The model under review builds one solid part; all positions refer to its coordinate system, in mm. A direction names the side the tool comes from. Coordinates: 2 decimals unless noted, no trailing zeros. Order: outer loops, then holes, each group sorted by start corner. A loop starts at its lowest first (then second) coordinate and runs counter-clockwise, first axis right, second up.
```python
from build123d import *

# Parameters (mm, degrees)
EXTRUDE_1_DEPTH     = 500
CUT_EXTRUDE_1_DEPTH = 165
SKETCH_4_R          = 20
SKETCH_4_R_2        = 9.341042427
SKETCH_4_R_3        = 10
EXTRUDE_2_DEPTH     = 30
SKETCH_5_R          = 8.254931616
SKETCH_5_R_2        = 9.226679221
EXTRUDE_3_DEPTH     = 30


with BuildPart() as part:
    # Эскиз2 → Бобышка-Вытянуть1 (new body)
    with BuildSketch(Plane.XY):
        with BuildLine():
            Line((-164, 0), (164, 0))
            Line((164, 0), (164, 281.346442364))
            ThreePointArc((164, 281.346442364), (158.142135624, 295.488577987), (144, 301.346442364))
            Line((144, 301.346442364), (128.648418925, 301.346442364))
            Line((128.648418925, 301.346442364), (102.483646542, 329.199264578))
            Line((102.483646542, 329.199264578), (-102.483646542, 329.199264578))
            Line((-102.483646542, 329.199264578), (-128.648418925, 301.346442364))
            Line((-128.648418925, 301.346442364), (-144, 301.346442364))
            ThreePointArc((-144, 301.346442364), (-158.142135624, 295.488577987), (-164, 281.346442364))
            Line((-164, 281.346442364), (-164, 0))
        make_face()
    extrude(amount=EXTRUDE_1_DEPTH)

    # Эскиз3 → Вырез-Вытянуть1 (cut, symmetric)
    with BuildSketch(Plane(origin=(0, 0, 0), x_dir=(0, 0, -1), z_dir=(1, 0, 0))):
        Polygon((-463.138471818, 344.733431976), (-500, 301.346442364), (-514.613262102, 301.346442364), (-514.613262102, 363.370856045), (0, 363.370856045), (0, 301.346442364), (-40.69019293, 344.733431976), (-73.527559146, 339.458620278), (-40.69019293, 301.346442364), (-469.350946507, 301.346442364), (-431.238768593, 339.458620278), align=None)
    extrude(amount=CUT_EXTRUDE_1_DEPTH, both=True, mode=Mode.SUBTRACT)

    # Эскиз4 → Бобышка-Вытянуть2 (add)
    with BuildSketch(Plane.XY.offset(500)):
        with Locations((-110, 47.069313646)):
            Circle(SKETCH_4_R)
        with Locations((-60, 47.069313646)):
            Circle(SKETCH_4_R_2)
        with Locations((110.509329497, 47.069313646)):
            Circle(SKETCH_4_R)
        with Locations((-35, 250)):
            Circle(SKETCH_4_R_3)
        with Locations((-55, 220)):
            Circle(SKETCH_4_R_3)
        with Locations((-15, 220)):
            Circle(SKETCH_4_R_3)
        with Locations((25, 220)):
            Circle(SKETCH_4_R_3)
        with Locations((65, 220)):
            Circle(SKETCH_4_R_3)
        with Locations((5, 250)):
            Circle(SKETCH_4_R_3)
        with Locations((45, 250)):
            Circle(SKETCH_4_R_3)
    extrude(amount=EXTRUDE_2_DEPTH)

    # Эскиз5 → Бобышка-Вытянуть3 (add)
    with BuildSketch(Plane(origin=(0, 0, 0), x_dir=(-1, 0, 0), z_dir=(0, 0, -1))):
        with Locations((-12.302238961, 29.934052236)):
            Circle(SKETCH_5_R)
        with Locations((-73.813433765, 29.934052236)):
            Circle(SKETCH_5_R_2)
    extrude(amount=EXTRUDE_3_DEPTH)


solid = part.part
```
(1) Machinability: for faces 1 (the face through (3.698, 259.915, 514.79)), 2 (the face through (13.38, 38.12, -14.79)), 3 (the face through (12, 30, -30)), which of the approach directions +Z, -Z, +X, -X, +Y, -Y give a long, thin tool a straight path to every point of the face, cutting with its end or side? Answer none if there is none.
A:
face 1: +Z
face 2: -Z
face 3: -Z, +X, -X, +Y, -Y
(2) For pin 1 Ø1.5 at (x, y) = (89.5, 250.5) entering from -Z; pin 2 Ø1 at (x, y) = (66, 178.5) entering from +Z; pin 3 Ø10 at (x, z) = (-113.5, 164) entering from +Y; pin 4 Ø3 at (x, z) = (-127.5, 67.5) entering from -Y, all flat-tipped, find the tip position at first contact; note any pin that passes through.
A:
pin 1: stops at z = 0
pin 2: stops at z = 500
pin 3: stops at y = 301.35
pin 4: stops at y = 0
(3) We need section C-C, the plane z = 369. Write out the cut boundary in (x, y).
A:
outline: (-164, 0) - (164, 0) - (164, 281.35) arc R20 ccw to (144, 301.35) - (-144, 301.35) arc R20 ccw to (-164, 281.35) - close
(4) Wall thickness on probe 1 along Z at (x, y) = (-132.5, 274); probe 2 along Y at (x, z) = (-41, 289.5); probe 3 along Z at (x, y) = (-7, 302.5): over which ranges is each line inside the solid? List them lowest first.
A:
probe 1: z = 0 to 500
probe 2: y = 0 to 301.35
probe 3: z = 1.08 to 41.68, 468.2 to 499.02
(5) We need section D-D, the plane x = -110. Write out the cut boundary in (y, z).
A:
outline: (0, 0) - (301.35, 0) - (321.2, 18.62) - (321.2, 57.79) - (301.35, 40.69) - (301.35, 469.35) - (321.2, 449.5) - (321.2, 483.13) - (301.35, 500) - (67.07, 500) - (67.07, 530) - (27.07, 530) - (27.07, 500) - (0, 500) - close
(6) Draft analysis for pull direction X (two halves, no side actions). For faces 4 (the face through (43.698, 259.915, 514.79)), 5 (the face through (1.8, 315.1, 12.9)), 6 (the face through (-115.38, 315.47, 31.89)), state which applies: released by +X, released by -X, zero draft, split by the parting line, or undercut.
A:
face 4: undercut
face 5: zero draft
face 6: released by -X
(7) We need section B-B, the plane x = -15. Write out the cut boundary in (y, z), and give its area (3 significant figures).
A:
outline: (0, 0) - (301.35, 0) - (329.2, 26.12) - (329.2, 64.69) - (301.35, 40.69) - (301.35, 469.35) - (329.2, 441.5) - (329.2, 476.34) - (301.35, 500) - (230, 500) - (230, 530) - (210, 530) - (210, 500) - (0, 500) - close
area: 153,000 mm2
(8) We need section A-A, the plane y = 220. Write out the cut boundary in (x, z).
A:
outline: (-164, 0) - (164, 0) - (164, 500) - (75, 500) - (75, 530) - (55, 530) - (55, 500) - (35, 500) - (35, 530) - (15, 530) - (15, 500) - (-5, 500) - (-5, 530) - (-25, 530) - (-25, 500) - (-45, 500) - (-45, 530) - (-65, 530) - (-65, 500) - (-164, 500) - close
